```python
from build123d import *

# Parameters (mm, degrees)
EXTRUDE_THIN1_DEPTH = 15
SKETCH5_W           = 30
SKETCH5_H           = 10
BOSS_EXTRUDE2_DEPTH = 160
FILLET15_R          = 5


with BuildPart() as part:
    # Sketch2 → Extrude-Thin1 (new, symmetric)
    with BuildSketch(Plane.XY):
        with BuildLine():
            ThreePointArc((166.330603598, 33.062927418), (160.12783844, 28.366835098), (152.36969162, 28.948845927))
            Line((152.36969162, 28.948845927), (0, 100))
            Line((0, 100), (0, 0))
            Line((0, 0), (150, 0))
            Line((150, 0), (150, 10))
            Line((150, 10), (10, 10))
            Line((10, 10), (10, 84.303144229))
            Line((10, 84.303144229), (148.143509003, 19.885768057))
            ThreePointArc((148.143509003, 19.885768057), (162.954516568, 18.774656473), (174.796159143, 27.73992363))
            Line((174.796159143, 27.73992363), (166.330603598, 33.062927418))
        make_face()
    extrude_thin1 = extrude(amount=EXTRUDE_THIN1_DEPTH, both=True)

    # Sketch5 → Boss-Extrude2 (add)
    with BuildSketch(Plane.XY.offset(15)):
        with Locations((165, 5)):
            Rectangle(SKETCH5_W, SKETCH5_H)
    extrude(amount=-BOSS_EXTRUDE2_DEPTH)

    # Mirror1: Extrude-Thin1 across plane
    add(extrude_thin1.mirror(Plane.XY.offset(-65)))

    # Fillet15
    fillet15_edges = [part.edges().sort_by_distance(p)[0] for p in [
        (0, 100, 0),
        (0, 100, -130),
        (174.796159143, 27.73992363, -130),
        (166.330603598, 33.062927418, -130),
        (10, 10, -130),
        (10, 84.303144229, -130),
        (10, 84.303144229, 0),
        (10, 10, 0),
        (174.796159143, 27.73992363, 0),
        (166.330603598, 33.062927418, 0),
    ]]
    fillet(fillet15_edges, radius=FILLET15_R - 0.0001)  # a hair under: the kernel refuses the full size


solid = part.part
```
Work out the finished part from the listing and answer in its coordinate system (mm). A direction names the side the tool comes from. Give positions to 0.01 mm unless a question says otherwise; leave off trailing zeros. Order: outer loops, then holes, each group sorted by start corner. A loop starts at its lowest first (then second) coordinate and runs counter-clockwise, first axis right, second up. Notation, with made-up numbers: (47.25, 1) -> (84.25, 1) arc R18 cw to (84.25, 19) -> close; hole circle Ø8 at (-0.75, -17.5). An arc over 180 degrees is marked (long way). Answer as CSV lines item,"result". Start each with the question number.
(1) Section A-A, the plane y = 73 is taken. Write down the section's boundary in (x, z).
(2) Consider line 1 along Z through (x, y) = (54, 4); line 2 along Y through (x, z) = (70.5, -3.5); line 3 along Y through (x, z) = (58, 8). Determine where each line is inside the solid, lowest interval first.
(3) Section C-C, the plane x = 66.5 is taken. Write down the section's boundary in (y, z).
(4) Each of these flat-tipped pins is pushed along its axis until it touches: pin 1 Ø8 at (y, z) = (7.5, -50.5) entering from -X; pin 2 Ø6 at (x, z) = (68, -115.5) entering from +Y; pin 3 Ø2 at (x, y) = (98, 40.5) entering from +Z; pin 4 Ø15 at (y, z) = (41, 1.5) entering from +X. Where does it stop, or does it pass through?
(5) Section D-D, the plane z = -55 is taken. Write down the section's boundary in (x, y).
(6) Which of the six approach directions +Z, -Z, +X, -X, +Y, -Y give full straight-line access (tool end or side, diameter ignored) to faces 1 (the flat face through (180, 5, -64)), 2 (the flat face through (10, 45, -130)), 3 (the flat face through (154, 10, -66))?
(7) For a pull along X with two mould halves and no side action, classify faces 4 (the flat face through (83, 52, -145)), 5 (the cylindrical face through (158.51, 28.02, -130.21)), 6 (the flat face through (0, 47, 0)) as released by +X, released by -X, zero draft, split by the parting line, or undercut.
Entries:
1,outline,"(0, -145) -> (10, -145) -> (10, -115) -> (0, -115) -> close; (0, -15) -> (10, -15) -> (10, 15) -> (0, 15) -> close; (34.24, -145) -> (57.9, -145) -> (57.9, -115) -> (34.24, -115) -> close; (34.24, -15) -> (57.9, -15) -> (57.9, 15) -> (34.24, 15) -> close"
2,line 1,"-145 to -115, -15 to 15"
2,line 2,"0 to 10, 56.09 to 67.13"
2,line 3,"0 to 10, 61.92 to 72.95"
3,outline,"(0, -145) -> (10, -145) -> (10, -115) -> (0, -115) -> close; (0, -15) -> (10, -15) -> (10, 15) -> (0, 15) -> close; (57.96, -145) -> (68.99, -145) -> (68.99, -115) -> (57.96, -115) -> close; (57.96, -15) -> (68.99, -15) -> (68.99, 15) -> (57.96, 15) -> close"
4,pin 1,"x = 150"
4,pin 2,"y = 69.69"
4,pin 3,"through"
4,pin 4,"x = 142.61"
5,outline,"(150, 0) -> (180, 0) -> (180, 10) -> (150, 10) -> close"
6,face 1,"+Z, -Z, +X, +Y, -Y"
6,face 2,"+Z, -Z"
6,face 3,"+Z, -Z, +X"
7,face 4,"zero draft"
7,face 5,"undercut"
7,face 6,"released by -X"
